```python
from build123d import *

# Parameters (mm, degrees)
F0_W        = 11.2
F0_H        = 16.2
F0_W_2      = 7
F0_H_2      = 12
F1_DEPTH    = 14.1
F2_R        = 2
F3_DEPTH    = 2.1
F4_R        = 5
F5_T1_DEPTH = 19.1


# Not quite as in the source:
# - a fillet or chamfer that OpenCascade refuses, or shapes differently, is made with other operations: its cross-section is extruded or revolved along the edge and cut away or added


with BuildPart() as f1:
    # F0 (on Top) → F1 (new body)
    with BuildSketch(Plane.XY):
        Rectangle(F0_W, F0_H)
        Rectangle(F0_W_2, F0_H_2, mode=Mode.SUBTRACT)
    extrude(amount=F1_DEPTH)

    # F2 (on Top) → F3 (join)
    with BuildSketch(Plane.XY):
        Polygon((6, -18.0165283297), (18.5, -18.0165283297), (18.5, 0), (18.5, 18.0165283297), (-18.5, 18.0165283297), (-18.5, 0), (-18.5, -14.0165283297), (-18.5, -18.0165283297), (-14.5, -18.0165283297), (-6, -18.0165283297), (-6, -8.0361003056), (-3.5, -8.0361003056), (-3.5, -6), (-3.5, 0), (-3.5, 6), (3.5, 6), (3.5, 0), (3.5, -6), (3.5, -8.0361003056), (6, -8.0361003056), align=None)
        with Locations((-14.5, -14.0165283297)):
            Circle(F2_R, mode=Mode.SUBTRACT)
        with Locations((14.5, -14.0165283297)):
            Circle(F2_R, mode=Mode.SUBTRACT)
        with Locations((-14.5, 14.0165283297)):
            Circle(F2_R, mode=Mode.SUBTRACT)
        with Locations((14.5, 14.0165283297)):
            Circle(F2_R, mode=Mode.SUBTRACT)
    extrude(amount=-F3_DEPTH)

    # F4
    f4_edges = [f1.edges().sort_by_distance(p)[0] for p in [
        (-18.5, 18.016528, -1.05),
        (18.5, 18.016528, -1.05),
        (18.5, -18.016528, -1.05),
        (-18.5, -18.016528, -1.05),
        (6, -18.016528, -1.05),
        (-6, -18.016528, -1.05),
    ]]
    fillet(f4_edges, radius=F4_R)

    # F5: fillet of radius 2 on 4 edges, made by hand

    # F5_s2 → F5_t1 (cut)
    with BuildSketch(Plane.XY):
        with BuildLine():
            ThreePointArc((5.6, 6.1), (5.0142135624, 7.5142135624), (3.6, 8.1))
            Line((3.6, 8.1), (5.6, 8.1))
            Line((5.6, 8.1), (5.6, 6.1))
        make_face()
        with BuildLine():
            ThreePointArc((-3.6, 8.1), (-5.0142135624, 7.5142135624), (-5.6, 6.1))
            Line((-5.6, 6.1), (-5.6, 8.1))
            Line((-5.6, 8.1), (-3.6, 8.1))
        make_face()
        with BuildLine():
            ThreePointArc((5.6, -6.1), (5.0142135624, -7.5142135624), (3.6, -8.1))
            Line((3.6, -8.1), (5.6, -8.1))
            Line((5.6, -8.1), (5.6, -6.1))
        make_face()
        with BuildLine():
            ThreePointArc((-5.6, -6.1), (-5.0142135624, -7.5142135624), (-3.6, -8.1))
            Line((-3.6, -8.1), (-5.6, -8.1))
            Line((-5.6, -8.1), (-5.6, -6.1))
        make_face()
    extrude(amount=F5_T1_DEPTH, mode=Mode.SUBTRACT)


solid = f1.part
```
Model file for the job. Use its own axes, mm. A direction names the side the tool comes from. Give positions to 0.01 mm unless a question says otherwise; leave off trailing zeros. Order: outer loops, then holes, each group sorted by start corner. A loop starts at its lowest first (then second) coordinate and runs counter-clockwise, first axis right, second up.
1) Mould opens along X. For faces 1 (the cylindrical face through (-17, -16.59, -1.06)), 2 (the flat face through (-12, -18.017, -1)), 3 (the flat face through (6, -10, -1)), 4 (the flat face through (0, -6, 7)) say: +X half, -X half, draft (parallel to the pull), parting line (faces both ways), or undercut.
2) Saw through at B-B, the plane y = 4.5. Write the cut outline in (x, z), then the cut area to 3 significant figures.
3) Saw through at C-C, the plane z = 1.75. Write the cut outline in (x, y), then the cut area to 3 significant figures.
4) Wall check: probe 1 along X at (y, z) = (-3.5, 12); probe 2 along Y at (x, z) = (14.5, -1.6); probe 3 along Y at (x, z) = (2, 10.25). Give the ranges that are in metal, low to high.
5) Pin check, flat tips, straight feed: pin 1 (2 mm diameter, centred on x = 1, z = 10, fed in from +Y); pin 2 (1 mm diameter, centred on y = 3.5, z = 3, fed in from -X); pin 3 (1.5 mm diameter, centred on x = 7, z = 6, fed in from +Y); pin 4 (3.5 mm diameter, centred on y = -2, z = 4, fed in from +X). Stop position of each tip, or through.
6) Saw through at D-D, the plane x = -14.5. Write the cut outline in (y, z).
7) Saw through at A-A, the plane x = -0.5. Write the cut outline in (y, z).
8) 3-axis set-ups, long thin cutter, end or side, ignore diameter. For faces 5 (the flat face through (-5, -8.036, -1)), 6 (the flat face through (-6, -11, -1)), 7 (the cylindrical face through (-5.03, -7.5, 6.95)): which of +Z, -Z, +X, -X, +Y, -Y reach the whole face in a straight line?
Computed:
1. face 1: -X half
1. face 2: draft
1. face 3: undercut
1. face 4: undercut
2. outline: (-18.5, -2.1) - (-3.5, -2.1) - (-3.5, 14.1) - (-5.6, 14.1) - (-5.6, 0) - (-18.5, 0) - close; (3.5, -2.1) - (18.5, -2.1) - (18.5, 0) - (5.6, 0) - (5.6, 14.1) - (3.5, 14.1) - close
2. area: 122 mm2
3. outline: (-5.6, -6.1) arc R2 ccw to (-3.6, -8.1) - (3.6, -8.1) arc R2 ccw to (5.6, -6.1) - (5.6, 6.1) arc R2 ccw to (3.6, 8.1) - (-3.6, 8.1) arc R2 ccw to (-5.6, 6.1) - close; hole (-3.5, -6) - (3.5, -6) - (3.5, 6) - (-3.5, 6) - close
3. area: 94.0 mm2
4. probe 1: x = -5.6 to -3.5, 3.5 to 5.6
4. probe 2: y = -17.92 to -16.02, -12.02 to 12.02, 16.02 to 17.92
4. probe 3: y = -8.1 to -6, 6 to 8.1
5. pin 1: stops at y = 8.1
5. pin 2: stops at x = -5.6
5. pin 3: passes through
5. pin 4: stops at x = 5.6
6. outline: (-17.92, -2.1) - (-16.02, -2.1) - (-16.02, 0) - (-17.92, 0) - close; (-12.02, -2.1) - (12.02, -2.1) - (12.02, 0) - (-12.02, 0) - close; (16.02, -2.1) - (17.92, -2.1) - (17.92, 0) - (16.02, 0) - close
7. outline: (-8.1, 0) - (-6, 0) - (-6, 14.1) - (-8.1, 14.1) - close; (6, -2.1) - (18.02, -2.1) - (18.02, 0) - (8.1, 0) - (8.1, 14.1) - (6, 14.1) - close
8. face 5: -Z, -Y
8. face 6: +Z, -Z, -Y
8. face 7: +Z, -X, -Y
